Work out the finished part from the listing and answer in its coordinate system (mm). A direction names the side the tool comes from. Coordinates: 2 decimals unless noted, no trailing zeros. Order: outer loops, then holes, each group sorted by start corner. A loop starts at its lowest first (then second) coordinate and runs counter-clockwise, first axis right, second up. Notation, with made-up numbers: (85.25, -38) -> (99.25, -38) arc R14 cw to (99.25, -14) -> close; hole circle Ø5 at (78, -25). An arc over 180 degrees is marked (long way). Answer as CSV lines item,"result". Start each with the question number.
Item 1: Section B-B (x = -18.75) is taken. Write down the section's boundary in (y, z) (1 decimal), then the cut area to 3 significant figures.
Item 2: Straight lines are drawn through the part: L1, parallel to X at y = 1.75, z = 32; L2, parallel to Z at x = -21.75, y = -2.5; L3, parallel to Y at x = -31.5, z = 32.5 (3 decimals). For each, find the intervals that lie inside material, in ascending order.
Item 3: Each of these flat-tipped pins is pushed along its axis until it touches: pin 1 Ø1.7 at (x, z) = (-34.5, 58.5) entering from +Y; pin 2 Ø4.5 at (x, z) = (-25.5, 43) entering from +Y; pin 3 Ø1.3 at (x, z) = (-31, 39) entering from -Y (3 decimals); pin 4 Ø3.5 at (y, z) = (-1.5, 52.5) entering from -X. Where does it stop, or does it pass through?
Item 4: Section C-C (z = 5) is taken. Write down the section's boundary in (x, y).
Item 5: Section D-D (z = 41) is taken. Write down the section's boundary in (x, y) (3 decimals).
Item 6: Which of the six approach directions +Z, -Z, +X, -X, +Y, -Y give full straight-line access (tool end or side, diameter ignored) to faces 1 (the face through (-31.758, 2, 49)), 2 (the face through (-30, 3.175, 50)), 3 (the face through (-30, -3.175, 50)), 4 (the face through (-28, -0.127, 44))?
Item 7: Section A-A (z = 51.5) is taken. Write down the section's boundary in (x, y) (3 decimals), then the cut area to 3 significant figures.
```python
from build123d import *

# Parameters (mm, degrees)
F2_DEPTH = 4.445
F3_DEPTH = 0.127
F4_DEPTH = 3.175


with BuildPart() as f1:
    # F0 (on Front) → F1 (revolve)
    with BuildSketch(Plane.XZ):
        with BuildLine():
            Line((-26.645181, 19.392501), (-30.455181, 19.392501))
            Line((-30.455181, 19.392501), (-30.455181, 3.810044))
            ThreePointArc((-30.455181, 3.810044), (-27.767587, 2.700607), (-26.645181, 0.018404))
            Line((-26.645181, 0.018404), (-26.645181, 19.392501))
        make_face()
        with BuildLine():
            Line((-26.645181, 0.018404), (-30.455181, 0.018404))
            Line((-30.455181, 0.018404), (-30.455181, -3.810044))
            ThreePointArc((-30.455181, -3.810044), (-27.761072, -2.694108), (-26.645136, 0))
            ThreePointArc((-26.645136, 0), (-26.645147, 0.009202), (-26.645181, 0.018404))
        make_face()
        with BuildLine():
            ThreePointArc((-26.645181, 0.018404), (-27.767587, 2.700607), (-30.455181, 3.810044))
            Line((-30.455181, 3.810044), (-30.455181, 0.018404))
            Line((-30.455181, 0.018404), (-26.645181, 0.018404))
        make_face()
    revolve(axis=Axis((-30.455181, 0, 9.705453), (0, 0, -1)))

    # F0 (on Front) → F2 (join, symmetric)
    with BuildSketch(Plane.XZ):
        Polygon((-44.425181, 19.392501), (-34.265181, 19.392501), (-30.455181, 19.392501), (-26.645181, 19.392501), (-16.485181, 19.392501), (-16.485181, 25.742501), (-23.470181, 25.742501), (-29.15215, 25.742501), (-30.455181, 25.742501), (-31.758212, 25.742501), (-37.440181, 25.742501), (-44.425181, 25.742501), align=None)
    extrude(amount=F2_DEPTH, both=True)

    # F0 (on Front) → F3 (join, symmetric)
    with BuildSketch(Plane.XZ):
        with BuildLine():
            Line((-29.15215, 25.742501), (-23.470181, 25.742501))
            ThreePointArc((-23.470181, 25.742501), (-27.34467, 46.412762), (-26.645181, 67.431375))
            Line((-26.645181, 67.431375), (-29.15215, 70.919501))
            Line((-29.15215, 70.919501), (-29.15215, 25.742501))
        make_face()
        with BuildLine():
            ThreePointArc((-34.265181, 67.431375), (-33.565691, 46.412762), (-37.440181, 25.742501))
            Line((-37.440181, 25.742501), (-31.758212, 25.742501))
            Line((-31.758212, 25.742501), (-31.758212, 70.919501))
            Line((-31.758212, 70.919501), (-34.265181, 67.431375))
        make_face()
    extrude(amount=F3_DEPTH, both=True)

    # F0 (on Front) → F4 (join, symmetric)
    with BuildSketch(Plane.XZ):
        Polygon((-30.455181, 72.732501), (-30.455181, 25.742501), (-29.15215, 25.742501), (-29.15215, 70.919501), align=None)
        Polygon((-31.758212, 70.919501), (-31.758212, 25.742501), (-30.455181, 25.742501), (-30.455181, 72.732501), align=None)
    extrude(amount=F4_DEPTH, both=True)


solid = f1.part
```
Checked values:
1,outline,"(-4.4, 19.4) -> (4.4, 19.4) -> (4.4, 25.7) -> (-4.4, 25.7) -> close"
1,area,"56.5 mm^2"
2,L1,"x = -31.76 to -29.15"
2,L2,"z = 19.39 to 25.74"
2,L3,"y = -3.175 to 3.175"
3,pin 1,"passes through"
3,pin 2,"stops at y = 0.13"
3,pin 3,"stops at y = -3.175"
3,pin 4,"stops at x = -33.32"
4,outline,"circle Ø7.62 at (-30.46, 0)"
5,outline,"(-34.132, -0.127) -> (-31.758, -0.127) -> (-31.758, -3.175) -> (-29.152, -3.175) -> (-29.152, -0.127) -> (-26.778, -0.127) -> (-26.778, 0.127) -> (-29.152, 0.127) -> (-29.152, 3.175) -> (-31.758, 3.175) -> (-31.758, 0.127) -> (-34.132, 0.127) -> close"
6,face 1,"+Z, -X, +Y"
6,face 2,"+Z, +X, -X, +Y"
6,face 3,"+Z, +X, -X, -Y"
6,face 4,"+Z, +X, -Y"
7,outline,"(-33.313, -0.127) -> (-31.758, -0.127) -> (-31.758, -3.175) -> (-29.152, -3.175) -> (-29.152, -0.127) -> (-27.597, -0.127) -> (-27.597, 0.127) -> (-29.152, 0.127) -> (-29.152, 3.175) -> (-31.758, 3.175) -> (-31.758, 0.127) -> (-33.313, 0.127) -> close"
7,area,"17.3 mm^2"
